Could you check a few things on this model? Use its own coordinates, in mm. A direction names the side the tool comes from. Give positions to 0.01 mm unless a question says otherwise; leave off trailing zeros. Loops run counter-clockwise (first coordinate to the right, second up) from the corner with the lowest first, then second, coordinate; pieces in that order, holes last. Notation, with made-up numbers: (30, 42) - (39, 42) arc R26 ccw to (39, 79) - close; hole circle Ø2 at (-32.5, 46.25). An arc over 180 degrees is marked (long way). One line per item, written item: value. Start each with the question number.
Q1. I want a section at A-A (y = -20). Please give me the cut outline in (x, z), then the cut area to 3 significant figures.
Q2. I'm going to push flat-ended pins straight in: P1, Ø5, axis at x = 12, y = -7, coming from the +Z side; P2, Ø3, axis at y = -2.5, z = -2.5, coming from the -X side; P3, Ø11, axis at y = -5.5, z = -2.5, coming from the +X side; P4, Ø4, axis at x = 86.5, y = -13, coming from the -Z side. Where does each tip first touch, or does it pass through?
Q3. If I drill on line 1 (Z direction, x = 0, y = -6.25); line 2 (Z direction, x = 276, y = -3), over which ranges is the centre line in solid material (lowest first)? Write a range as from..to.
Q4. I want a section at C-C (z = 98). Please give me the cut outline in (x, y), then the cut area to 3 significant figures.
Q5. If we mould it in two halves opening along Z, with no side actions, what happens to faces 1 (the face through (-69.188, -4.93, 70.784)), 2 (the face through (-91.87, -4.93, 74.62)), 3 (the face through (189, -10, 393))? For each: released by +Z, released by -Z, zero draft, split by the parting line, or undercut.
Q6. For faces 4 (the face through (283.59, -4.93, 474.51)), 5 (the face through (285.72, -4.93, 450.19)), which set-ups out of +Z, -Z, +X, -X, +Y, -Y let a thin tool reach every point of the face, with its end or its side?
Q7. I want a section at B-B (x = 574.5). Please give me the cut outline in (y, z), then the cut area to 3 significant figures.
```python
from build123d import *

# Parameters (mm, degrees)
F0_W     = 131.7172
F0_H     = 20
F0_R     = 5
F1_DEPTH = 10
F2_R     = 5
F3_DEPTH = 50
F5_DEPTH = 10
F7_DEPTH = 10


with BuildPart() as f1:
    # F0 (on Front) → F1 (new body)
    with BuildSketch(Plane.XZ):
        Rectangle(F0_W, F0_H)
        Circle(F0_R, mode=Mode.SUBTRACT)
    extrude(amount=F1_DEPTH)

    # F2 (on face) → F3 (join)
    with BuildSketch(Plane.XZ.offset(10)):
        with Locations((-45.8586, 0)):
            Circle(F2_R)
        with Locations((45.8586, 0)):
            Circle(F2_R)
    extrude(amount=F3_DEPTH)

    # F4 (on Front) → F5 (join)
    with BuildSketch(Plane.XZ):
        Polygon((-117.161621, 144.11349), (-65.8586, 3.159597), (-47.064747, 10), (-98.367769, 150.953893), align=None)
    extrude(amount=F5_DEPTH)

    # F6 (on Front) → F7 (join)
    with BuildSketch(Plane.XZ):
        Polygon((661.248798, 791.401947), (-104.795645, 148.614338), (-91.939893, 133.293449), (674.104551, 776.081058), align=None)
    extrude(amount=F7_DEPTH)


solid = f1.part
```
Worked answers:
1. outline: circle Ø10 at (-45.86, 0); circle Ø10 at (45.86, 0)
1. area: 157 mm²
2. P1: stops at z = 248.72
2. P2: stops at x = -65.86
2. P3: stops at x = 65.86
2. P4: passes through
3. line 1: z = -10..-5, 5..10, 210.44..236.55
3. line 2: z = 442.03..468.14
4. outline: (-100.38, -10) - (-79.09, -10) - (-79.09, 0) - (-100.38, 0) - close
4. area: 213 mm²
5. face 1: undercut
5. face 2: released by -Z
5. face 3: zero draft
6. face 4: +Z, -X, +Y, -Y
6. face 5: +X, +Y, -Y
7. outline: (-10, 692.5) - (0, 692.5) - (0, 718.61) - (-10, 718.61) - close
7. area: 261 mm²
